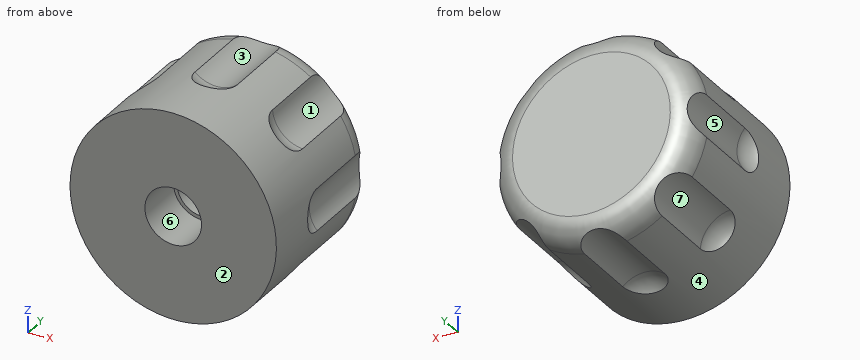
```python
from build123d import *

# Parameters (mm, degrees)
SKETCH1_R               = 12.75
BOSS_EXTRUDE1_DEPTH     = 20
CUT_EXTRUDE1_DEPTH      = 27.928145127
CUT_EXTRUDE1_DEPTH_BACK = 18.3
SKETCH2_R               = 3.05
SKETCH3_R               = 3.5
CUT_EXTRUDE2_DEPTH      = 6
FILLET1_R               = 3
SKETCH5_R               = 4
CUT_EXTRUDE3_DEPTH      = 14
FILLET3_R               = 3


with BuildPart() as part:
    # Sketch1 → Boss-Extrude1 (new body)
    with BuildSketch(Plane(origin=(0, 0, 0), x_dir=(1, 0, 0), z_dir=(0, 1, 0))):
        with Locations(Location((0, 0, 0), (0, 0, 270))):
            Circle(SKETCH1_R)
    extrude(amount=BOSS_EXTRUDE1_DEPTH)

    # Sketch2 → Cut-Extrude1 (cut, two sides: drawn at the far end of the back side and taken through both)
    with BuildSketch(Plane.XZ.offset(-CUT_EXTRUDE1_DEPTH_BACK)):
        with Locations(Location((0, 0, 0), (0, 0, 90))):
            Circle(SKETCH2_R)
    extrude(amount=CUT_EXTRUDE1_DEPTH + CUT_EXTRUDE1_DEPTH_BACK, mode=Mode.SUBTRACT)

    # Sketch3 → Cut-Extrude2 (cut)
    with BuildSketch(Plane.XZ):
        with Locations(Location((0, 0, 0), (0, 0, 270))):
            Circle(SKETCH3_R)
    extrude(amount=-CUT_EXTRUDE2_DEPTH, mode=Mode.SUBTRACT)

    # Fillet1
    fillet1_edges = [part.edges().sort_by_distance(p)[0] for p in [
        (0, 20, -12.75),
    ]]
    fillet(fillet1_edges, radius=FILLET1_R)

    # Sketch5 → Cut-Extrude3 (cut)
    with BuildSketch(Plane(origin=(0, 20, 0), x_dir=(1, 0, 0), z_dir=(0, 1, 0))):
        with Locations((0, 15.5)):
            Circle(SKETCH5_R)
        with Locations((10.960155108, 10.960155108)):
            Circle(SKETCH5_R)
        with Locations((15.5, 0)):
            Circle(SKETCH5_R)
        with Locations((10.960155108, -10.960155108)):
            Circle(SKETCH5_R)
        with Locations((0, -15.5)):
            Circle(SKETCH5_R)
        with Locations((-10.960155108, -10.960155108)):
            Circle(SKETCH5_R)
        with Locations((-15.5, 0)):
            Circle(SKETCH5_R)
        with Locations((-10.960155108, 10.960155108)):
            Circle(SKETCH5_R)
    extrude(amount=-CUT_EXTRUDE3_DEPTH, mode=Mode.SUBTRACT)

    # Fillet3
    # the kernel refuses this fillet: 3 mm, written as the material it adds along each edge
    with BuildSketch(Plane(origin=(0, 6, 15.5), x_dir=(0.5240999982324142, 0, 0.8516567335803691), z_dir=(-0.8516567335803691, 0, 0.5240999982324142))) as fillet3_piece_1_section:
        with BuildLine():
            CenterArc((4 - FILLET3_R, FILLET3_R), FILLET3_R, 270, 90)
            Line((4 - FILLET3_R, 0), (4, 0))
            Line((4, 0), (4, FILLET3_R))
        make_face()
    fillet3_piece_1 = revolve(axis=Axis((0, 6, 15.5), (0, 1, 0)), revolution_arc=296.784649365, mode=Mode.PRIVATE)
    fillet3_piece_1 = fillet3_piece_1 & Plane(origin=(0, 6.906503108, 0), x_dir=(0, 0, 1), z_dir=(0, -1, 0)) * Cylinder(12.75, 17, mode=Mode.PRIVATE)
    add(fillet3_piece_1)
    with BuildSketch(Plane(origin=(-10.960155108, 6, 10.960155108), x_dir=(-0.2316175887878651, 0, 0.9728069143278617), z_dir=(-0.9728069143278617, 0, -0.2316175887878651))) as fillet3_piece_2_section:
        with BuildLine():
            CenterArc((4 - FILLET3_R, FILLET3_R), FILLET3_R, 270, 90)
            Line((4, FILLET3_R), (4, 0))
            Line((4, 0), (4 - FILLET3_R, 0))
        make_face()
    fillet3_piece_2 = revolve(axis=Axis((-10.960155108, 6, 10.960155108), (0, 1, 0)), revolution_arc=296.784649365, mode=Mode.PRIVATE)
    fillet3_piece_2 = fillet3_piece_2 & Plane(origin=(0, 6.906501973, 0), x_dir=(0, 0, 1), z_dir=(0, -1, 0)) * Cylinder(12.75, 16, mode=Mode.PRIVATE)
    add(fillet3_piece_2)
    with BuildSketch(Plane(origin=(-15.5, 6, 0), x_dir=(-0.8516567335803689, 0, -0.524099998232414), z_dir=(-0.524099998232414, 0, 0.8516567335803689))) as fillet3_piece_3_section:
        with BuildLine():
            CenterArc((4 - FILLET3_R, -FILLET3_R), FILLET3_R, 0, 90)
            Line((4, -FILLET3_R), (4, 0))
            Line((4, 0), (4 - FILLET3_R, 0))
        make_face()
    fillet3_piece_3 = revolve(axis=Axis((-15.5, 6, 0), (0, -1, 0)), revolution_arc=296.784649365, mode=Mode.PRIVATE)
    fillet3_piece_3 = fillet3_piece_3 & Plane(origin=(0, 6.90650195, 0), x_dir=(0, 0, 1), z_dir=(0, -1, 0)) * Cylinder(12.75, 16, mode=Mode.PRIVATE)
    add(fillet3_piece_3)
    with BuildSketch(Plane(origin=(-10.960155108, 6, -10.960155108), x_dir=(-0.9728069143278615, 0, -0.23161758878786548), z_dir=(0.23161758878786548, 0, -0.9728069143278615))) as fillet3_piece_4_section:
        with BuildLine():
            CenterArc((4 - FILLET3_R, FILLET3_R), FILLET3_R, 270, 90)
            Line((4, FILLET3_R), (4, 0))
            Line((4, 0), (4 - FILLET3_R, 0))
        make_face()
    fillet3_piece_4 = revolve(axis=Axis((-10.960155108, 6, -10.960155108), (0, 1, 0)), revolution_arc=296.784649365, mode=Mode.PRIVATE)
    fillet3_piece_4 = fillet3_piece_4 & Plane(origin=(0, 6.906501973, 0), x_dir=(0, 0, 1), z_dir=(0, -1, 0)) * Cylinder(12.75, 17, mode=Mode.PRIVATE)
    add(fillet3_piece_4)
    with BuildSketch(Plane(origin=(0, 6, -15.5), x_dir=(-0.5240999982324135, 0, -0.8516567335803694), z_dir=(0.8516567335803694, 0, -0.5240999982324135))) as fillet3_piece_5_section:
        with BuildLine():
            CenterArc((4 - FILLET3_R, FILLET3_R), FILLET3_R, 270, 90)
            Line((4, FILLET3_R), (4, 0))
            Line((4, 0), (4 - FILLET3_R, 0))
        make_face()
    fillet3_piece_5 = revolve(axis=Axis((0, 6, -15.5), (0, 1, 0)), revolution_arc=296.784649365, mode=Mode.PRIVATE)
    fillet3_piece_5 = fillet3_piece_5 & Plane(origin=(0, 6.906501973, 0), x_dir=(0, 0, 1), z_dir=(0, -1, 0)) * Cylinder(12.75, 16, mode=Mode.PRIVATE)
    add(fillet3_piece_5)
    with BuildSketch(Plane(origin=(10.960155108, 6, -10.960155108), x_dir=(0.2316175887878651, 0, -0.9728069143278617), z_dir=(0.9728069143278617, 0, 0.2316175887878651))) as fillet3_piece_6_section:
        with BuildLine():
            CenterArc((4 - FILLET3_R, FILLET3_R), FILLET3_R, 270, 90)
            Line((4, FILLET3_R), (4, 0))
            Line((4, 0), (4 - FILLET3_R, 0))
        make_face()
    fillet3_piece_6 = revolve(axis=Axis((10.960155108, 6, -10.960155108), (0, 1, 0)), revolution_arc=296.784649365, mode=Mode.PRIVATE)
    fillet3_piece_6 = fillet3_piece_6 & Plane(origin=(0, 6.906501973, 0), x_dir=(0, 0, 1), z_dir=(0, -1, 0)) * Cylinder(12.75, 16, mode=Mode.PRIVATE)
    add(fillet3_piece_6)
    with BuildSketch(Plane(origin=(15.5, 6, 0), x_dir=(0.8516567335803694, 0, -0.5240999982324135), z_dir=(0.5240999982324135, 0, 0.8516567335803694))) as fillet3_piece_7_section:
        with BuildLine():
            CenterArc((4 - FILLET3_R, FILLET3_R), FILLET3_R, 270, 90)
            Line((4, FILLET3_R), (4, 0))
            Line((4, 0), (4 - FILLET3_R, 0))
        make_face()
    fillet3_piece_7 = revolve(axis=Axis((15.5, 6, 0), (0, 1, 0)), revolution_arc=296.784649365, mode=Mode.PRIVATE)
    fillet3_piece_7 = fillet3_piece_7 & Plane(origin=(0, 6.906501973, 0), x_dir=(0, 0, 1), z_dir=(0, -1, 0)) * Cylinder(12.75, 17, mode=Mode.PRIVATE)
    add(fillet3_piece_7)
    with BuildSketch(Plane(origin=(10.960155108, 6, 10.960155108), x_dir=(0.9728069143278617, 0, 0.2316175887878651), z_dir=(-0.2316175887878651, 0, 0.9728069143278617))) as fillet3_piece_8_section:
        with BuildLine():
            CenterArc((4 - FILLET3_R, FILLET3_R), FILLET3_R, 270, 90)
            Line((4, FILLET3_R), (4, 0))
            Line((4, 0), (4 - FILLET3_R, 0))
        make_face()
    fillet3_piece_8 = revolve(axis=Axis((10.960155108, 6, 10.960155108), (0, 1, 0)), revolution_arc=296.784649365, mode=Mode.PRIVATE)
    fillet3_piece_8 = fillet3_piece_8 & Plane(origin=(0, 6.906501973, 0), x_dir=(0, 0, 1), z_dir=(0, -1, 0)) * Cylinder(12.75, 16, mode=Mode.PRIVATE)
    add(fillet3_piece_8)


solid = part.part
```
Part model, mm, in its own coordinate system. Face numbers are marked on the shaded views. A direction names the side the tool comes from. Round coordinates to 2 decimals unless told otherwise and drop trailing zeros. Write each loop counter-clockwise with the first axis right and the second up, starting at its lowest first coordinate (ties: lowest second). Pieces come first, ordered by that corner, then holes. Notation, with made-up numbers: (-28, -11) -> (-18, -11) arc R16 ccw to (-18, -3) -> close; hole circle Ø11 at (-37, 17.5). An arc over 180 degrees is marked (long way). Return JSON: item names as keys, results as strings. Group by question number.
Q1. Pin check, flat tips, straight feed: pin 1 (1 mm diameter, centred on y = 3, z = 6.5, fed in from +X); pin 2 (8 mm diameter, centred on y = 11.5, z = -2, fed in from -X); pin 3 (5 mm diameter, centred on x = 0.5, z = -0.5, fed in from -Y). Stop position of each tip, or through.
Q2. Saw through at B-B on y = 5.5. Write the cut outline in (x, z), plus the area to 3 significant figures.
Q3. Probe L1, parallel to X at y = 10.25, z = 0; L2, parallel to Y at x = -0.75, z = 0; L3, parallel to Y at x = 2.75, z = -1.75. List the from-to ranges inside material, lowest first. Write a range as [from, to].
Q4. Which spindle directions (+Z, -Z, +X, -X, +Y, -Y) get a long thin tool onto all of the face, cutting with end or side? Do the marked faces 5, 6 and 7. Say none if no direction does.
Q5. Mould opens along X. For the marked faces 1, 2, 3 and 4 say: pulls with the +X half, pulls with the -X half, needs draft (parallel to the pull), parting line crosses it, or undercut.
Q6. Saw through at A-A on y = 11.5. Write the cut outline in (x, z).
Answer:
{
 "1": {"pin 1": "x = 11.25", "pin 2": "x = -12.58", "pin 3": "y = 6"},
 "2": {"outline": "circle Ø25.5 at (0, 0); hole circle Ø7 at (0, 0)", "area": "472 mm2"},
 "3": {"L1": "[-11.5, -3.05], [3.05, 11.5]", "L2": "[18.3, 20]", "L3": "[6, 20]"},
 "4": {"face 5": "-X, +Y", "face 6": "-Y", "face 7": "-Z, -X, +Y"},
 "5": {"face 1": "pulls with the +X half", "face 2": "needs draft", "face 3": "undercut", "face 4": "parting line crosses it"},
 "6": {"outline": "(-12.48, -2.62) arc R12.75 ccw to (-10.68, -6.97) arc R4 cw to (-6.97, -10.68) arc R12.75 ccw to (-2.62, -12.48) arc R4 cw to (2.62, -12.48) arc R12.75 ccw to (6.97, -10.68) arc R4 cw to (10.68, -6.97) arc R12.75 ccw to (12.48, -2.62) arc R4 cw to (12.48, 2.62) arc R12.75 ccw to (10.68, 6.97) arc R4 cw to (6.97, 10.68) arc R12.75 ccw to (2.62, 12.48) arc R4 cw to (-2.62, 12.48) arc R12.75 ccw to (-6.97, 10.68) arc R4 cw to (-10.68, 6.97) arc R12.75 ccw to (-12.48, 2.62) arc R4 cw to start; hole circle Ø6.1 at (0, 0)"}
}
